from build123d import *

# Parameters (mm, degrees)
SKETCH_1_R             = 175
EXTRUDE_1_DEPTH        = 3
CUT_EXTRUDE_1_DEPTH    = 3
FILLET_1_R             = 5
FILLET_2_R             = 5
FILLET_3_R             = 5
SKETCH_5_R             = 1.5
CUT_EXTRUDE_4_DEPTH    = 3
SKETCH_6_R             = 1.5
CUT_EXTRUDE_5_DEPTH    = 3
SKETCH_7_W             = 30
SKETCH_7_H             = 108
CUT_EXTRUDE_6_DEPTH    = 3
SKETCH_8_R             = 1.5
CUT_EXTRUDE_7_DEPTH    = 3
SKETCH_9_R             = 1.5
CUT_EXTRUDE_8_DEPTH    = 10
SKETCH_10_R            = 1.6
CUT_EXTRUDE_9_DEPTH    = 10
SKETCH_11_W            = 15
SKETCH_11_H            = 30
CUT_EXTRUDE_10_DEPTH   = 10
SKETCH_12_R            = 1.5
CUT_EXTRUDE_11_DEPTH   = 4
SKETCH_13_R            = 1.5
CUT_EXTRUDE_12_DEPTH   = 4
PATTERN_LINEAR_1_COUNT = 2
PATTERN_LINEAR_1_PITCH = 73
SKETCH_14_R            = 1.5
CUT_EXTRUDE_14_DEPTH   = 4
SKETCH_17_R            = 1.5
CUT_EXTRUDE_15_DEPTH   = 4
SKETCH_18_R            = 1.5
CUT_EXTRUDE_16_DEPTH   = 4


with BuildPart() as part:
    # ｽｹｯﾁ1 → ﾎﾞｽ - 押し出し1 (new body)
    with BuildSketch(Plane.XY):
        Circle(SKETCH_1_R)
    extrude(amount=EXTRUDE_1_DEPTH)

    # ｽｹｯﾁ2 → ｶｯﾄ - 押し出し1 (cut)
    with BuildSketch(Plane.XY.offset(3)):
        with BuildLine():
            Line((-60, 115), (0, 115))
            Line((0, 115), (0, 175))
            ThreePointArc((0, 175), (-30.465194158, 172.327803749), (-60, 164.392822228))
            Line((-60, 164.392822228), (-60, 115))
        make_face()
        with BuildLine():
            Line((0, 175), (0, 115))
            Line((0, 115), (60, 115))
            Line((60, 115), (60, 164.392822228))
            ThreePointArc((60, 164.392822228), (30.465194158, 172.327803749), (0, 175))
        make_face()
        with BuildLine():
            Line((0, -175), (0, -115))
            Line((0, -115), (-60, -115))
            Line((-60, -115), (-60, -164.392822228))
            ThreePointArc((-60, -164.392822228), (-30.465194158, -172.327803749), (0, -175))
        make_face()
        with BuildLine():
            Line((60, -115), (0, -115))
            Line((0, -115), (0, -175))
            ThreePointArc((0, -175), (30.465194158, -172.327803749), (60, -164.392822228))
            Line((60, -164.392822228), (60, -115))
        make_face()
    extrude(amount=-CUT_EXTRUDE_1_DEPTH, mode=Mode.SUBTRACT)

    # ﾌｨﾚｯﾄ1
    fillet_1_edges = [part.edges().sort_by_distance(p)[0] for p in [
        (-60, 164.392822228, 1.5),
    ]]
    fillet(fillet_1_edges, radius=FILLET_1_R)

    # ﾌｨﾚｯﾄ2
    fillet_2_edges = [part.edges().sort_by_distance(p)[0] for p in [
        (-60, 115, 1.5),
        (60, 164.392822228, 1.5),
        (60, 115, 1.5),
    ]]
    fillet(fillet_2_edges, radius=FILLET_2_R)

    # ﾌｨﾚｯﾄ3
    fillet_3_edges = [part.edges().sort_by_distance(p)[0] for p in [
        (-60, -115, 1.5),
        (60, -115, 1.5),
        (60, -164.392822228, 1.5),
        (-60, -164.392822228, 1.5),
    ]]
    fillet(fillet_3_edges, radius=FILLET_3_R)

    # ｽｹｯﾁ5 → ｶｯﾄ - 押し出し4 (cut)
    with BuildSketch(Plane.XY.offset(3)):
        with Locations((-100, -115)):
            Circle(SKETCH_5_R)
        with Locations((100, -115)):
            Circle(SKETCH_5_R)
        with Locations((100, 115)):
            Circle(SKETCH_5_R)
        with Locations((-100, 115)):
            Circle(SKETCH_5_R)
    extrude(amount=-CUT_EXTRUDE_4_DEPTH, mode=Mode.SUBTRACT)

    # ｽｹｯﾁ6 → ｶｯﾄ - 押し出し5 (cut)
    with BuildSketch(Plane.XY.offset(3)):
        with Locations((-60, 54)):
            Circle(SKETCH_6_R)
        with Locations((60, 54)):
            Circle(SKETCH_6_R)
        with Locations((-60, -54)):
            Circle(SKETCH_6_R)
        with Locations((60, -54)):
            Circle(SKETCH_6_R)
    extrude(amount=-CUT_EXTRUDE_5_DEPTH, mode=Mode.SUBTRACT)

    # ｽｹｯﾁ7 → ｶｯﾄ - 押し出し6 (cut)
    with BuildSketch(Plane.XY.offset(3)):
        with Locations((-85, 0)):
            Rectangle(SKETCH_7_W, SKETCH_7_H)
    extrude(amount=-CUT_EXTRUDE_6_DEPTH, mode=Mode.SUBTRACT)

    # ｽｹｯﾁ8 → ｶｯﾄ - 押し出し7 (cut)
    with BuildSketch(Plane.XY.offset(3)):
        with Locations((-115, -67)):
            Circle(SKETCH_8_R)
        with Locations((-116.822468618, 0)):
            Circle(SKETCH_8_R)
        with Locations((-115, 67)):
            Circle(SKETCH_8_R)
    extrude(amount=-CUT_EXTRUDE_7_DEPTH, mode=Mode.SUBTRACT)

    # ｽｹｯﾁ9 → ｶｯﾄ - 押し出し8 (cut)
    with BuildSketch(Plane.XY.offset(3)):
        with Locations((-65, 37)):
            Circle(SKETCH_9_R)
        with Locations((20, 41)):
            Circle(SKETCH_9_R)
        with Locations((-65, -38)):
            Circle(SKETCH_9_R)
        with Locations((20, -40)):
            Circle(SKETCH_9_R)
    extrude(amount=-CUT_EXTRUDE_8_DEPTH, mode=Mode.SUBTRACT)

    # ｽｹｯﾁ10 → ｶｯﾄ - 押し出し9 (cut)
    with BuildSketch(Plane.XY.offset(3)):
        with Locations((111.643659725, -125.921059639)):
            Circle(SKETCH_10_R)
        with Locations((122.679794489, -115.037952538)):
            Circle(SKETCH_10_R)
        with Locations((168, 7.75)):
            Circle(SKETCH_10_R)
        with Locations((168, -7.75)):
            Circle(SKETCH_10_R)
        with Locations((111.56768007, 125.844011632)):
            Circle(SKETCH_10_R)
        with Locations((122.679794489, 115.037952538)):
            Circle(SKETCH_10_R)
    extrude(amount=-CUT_EXTRUDE_9_DEPTH, mode=Mode.SUBTRACT)

    # ｽｹｯﾁ11 → ｶｯﾄ - 押し出し10 (cut)
    with BuildSketch(Plane.XY.offset(3)):
        with Locations((81.317279836, 81.317279836)):
            Rectangle(SKETCH_11_W, SKETCH_11_H)
        with Locations((81.317279836, -81.317279836)):
            Rectangle(SKETCH_11_W, SKETCH_11_H)
    extrude(amount=-CUT_EXTRUDE_10_DEPTH, mode=Mode.SUBTRACT)

    # ｽｹｯﾁ12 → ｶｯﾄ - 押し出し11 (cut, through all)
    with BuildSketch(Plane.XY.offset(3)):
        with Locations((139.4, 10.5)):
            Circle(SKETCH_12_R)
        with Locations((139.4, -10.5)):
            Circle(SKETCH_12_R)
    extrude(amount=-CUT_EXTRUDE_11_DEPTH, mode=Mode.SUBTRACT)

    # ｽｹｯﾁ13 → ｶｯﾄ - 押し出し12 (cut, through all)
    with BuildSketch(Plane.XY.offset(3)):
        with Locations((89.692125231, 10)):
            Circle(SKETCH_13_R)
        with Locations((89.692125231, 63)):
            Circle(SKETCH_13_R)
        with Locations((-22.988418993, 63)):
            Circle(SKETCH_13_R)
        with Locations((-22.988418993, 10)):
            Circle(SKETCH_13_R)
        with Locations((116.692125231, 36.5)):
            Circle(SKETCH_13_R)
    cut_extrude_12 = extrude(amount=-CUT_EXTRUDE_12_DEPTH, mode=Mode.SUBTRACT)

    # 直線ﾊﾟﾀｰﾝ1: ｶｯﾄ - 押し出し12 ×2
    with Locations(*[(0, -i * PATTERN_LINEAR_1_PITCH, 0) for i in range(1, PATTERN_LINEAR_1_COUNT)]):
        add(cut_extrude_12, mode=Mode.SUBTRACT)

    # ｽｹｯﾁ14 → ｶｯﾄ - 押し出し14 (cut, through all)
    with BuildSketch(Plane.XY.offset(3)):
        with Locations((108.817279836, 89.5)):
            Circle(SKETCH_14_R)
        with Locations((108.817279836, 60)):
            Circle(SKETCH_14_R)
    extrude(amount=-CUT_EXTRUDE_14_DEPTH, mode=Mode.SUBTRACT)

    # ｽｹｯﾁ17 → ｶｯﾄ - 押し出し15 (cut, through all)
    with BuildSketch(Plane.XY.offset(3)):
        with Locations((108.817279836, -60)):
            Circle(SKETCH_17_R)
        with Locations((108.817279836, -89.5)):
            Circle(SKETCH_17_R)
    extrude(amount=-CUT_EXTRUDE_15_DEPTH, mode=Mode.SUBTRACT)

    # ｽｹｯﾁ18 → ｶｯﾄ - 押し出し16 (cut, through all)
    with BuildSketch(Plane.XY.offset(3)):
        with Locations((-124.610636376, 31.75)):
            Circle(SKETCH_18_R)
        with Locations((-124.610636376, -31.75)):
            Circle(SKETCH_18_R)
    extrude(amount=-CUT_EXTRUDE_16_DEPTH, mode=Mode.SUBTRACT)


solid = part.part
The listing builds one solid part. Answer for the finished solid, in the listing's coordinates (mm). Give positions to 0.01 mm unless a question says otherwise; leave off trailing zeros. Loops run counter-clockwise (first coordinate to the right, second up) from the corner with the lowest first, then second, coordinate; pieces in that order, holes last. Notation, with made-up numbers: (56.25, -30) - (74.25, -30) arc R27 ccw to (74.25, 3) - close; hole circle Ø3 at (-1.5, -31.5). An arc over 180 degrees is marked (long way). Answer as a JSON object with one key per item and string values.
1. A cutting plane is placed at D-D (z = 2.35). Give the number of separate pieces and of enclosed holes in the cut face, then the cut area to 3 significant figures.
Determined:
{"separate pieces": "1", "enclosed holes": "42", "area": "78,200 mm²"}
2. Find the intervals of material crossed by L1, parallel to Y at x = -65, z = 2.3; L2, parallel to Y at x = 20, z = 1.2; L3, parallel to X at y = 77, z = 0.3, in increasing order. Write a range as [from, to].
Determined:
{"L1": "[-162.08, -39.5], [-36.5, 35.5], [38.5, 162.08]", "L2": "[-115, -41.5], [-38.5, 39.5], [42.5, 115]", "L3": "[-157.15, 73.82], [88.82, 157.15]"}
3. A cutting plane is placed at A-A (y = -78). Write down the section's boundary in (x, z).
Determined:
{"outline": "(-156.66, 0) - (73.82, 0) - (73.82, 3) - (-156.66, 3) - close; (88.82, 0) - (156.66, 0) - (156.66, 3) - (88.82, 3) - close"}
4. A cutting plane is placed at B-B (y = -133). Write down the section's boundary in (x, z).
Determined:
{"outline": "(-113.74, 0) - (-60, 0) - (-60, 3) - (-113.74, 3) - close; (60, 0) - (113.74, 0) - (113.74, 3) - (60, 3) - close"}
5. A cutting plane is placed at C-C (x = -30). Write down the section's boundary in (y, z).
Determined:
{"outline": "(-115, 0) - (115, 0) - (115, 3) - (-115, 3) - close"}
6. Flat-ended cylindrical pins translate along their axes: pin 1 Ø3.5 at (x, y) = (20, 41) entering from -Z; pin 2 Ø1.5 at (y, z) = (137, 1.5) entering from +X; pin 3 Ø1.5 at (x, z) = (79.5, 1.5) entering from +Y; pin 4 Ø0.9 at (y, z) = (77, 1.5) entering from +X. Find the tip coordinate at first contact, or state that the pin passes through.
Determined:
{"pin 1": "z = 0", "pin 2": "x = 109.82", "pin 3": "y = 156.28", "pin 4": "x = 157.37"}
